```python
from build123d import *

# Parameters (mm, degrees)
SKETCH1_W           = 98
SKETCH1_H           = 65
BOSS_EXTRUDE1_DEPTH = 5
SKETCH2_W           = 16
SKETCH2_H           = 10
CUT_EXTRUDE1_DEPTH  = 15


with BuildPart() as part:
    # Sketch1 → Boss-Extrude1 (new body)
    with BuildSketch(Plane.XY):
        with Locations((49, -32.5)):
            Rectangle(SKETCH1_W, SKETCH1_H)
    extrude(amount=BOSS_EXTRUDE1_DEPTH)

    # Sketch2 → Cut-Extrude1 (cut)
    with BuildSketch(Plane.XY.offset(5)):
        Polygon((82, -45), (82, -40), (82, -35), (66, -35), (66, -45), align=None)
        with Locations((24, -40)):
            Rectangle(SKETCH2_W, SKETCH2_H)
    extrude(amount=-CUT_EXTRUDE1_DEPTH, mode=Mode.SUBTRACT)


solid = part.part
```
Design review of the part built by this model. Coordinates are the model's own, in mm. A direction names the side the tool comes from. Round coordinates to 2 decimals unless told otherwise and drop trailing zeros. Write each loop counter-clockwise with the first axis right and the second up, starting at its lowest first coordinate (ties: lowest second). Pieces come first, ordered by that corner, then holes. Notation, with made-up numbers: (-27, 27) -> (-10, 27) arc R28 cw to (-10, 51) -> close; hole circle Ø8 at (-13.75, -30.75). An arc over 180 degrees is marked (long way). Write item = value, one per line. Start each with the question number.
1) Tool access review of faces 1 (the face through (48, -32, 0)), 2 (the face through (24, -35, 3)): name each direction out of +Z, -Z, +X, -X, +Y, -Y from which nothing blocks a thin tool from reaching the whole face with its end or side.
2) Wall thickness on probe 1 along X at (y, z) = (-42.5, 2.5); probe 2 along Y at (x, z) = (80, 4.05): over which ranges is each line inside the solid? List them lowest first. Write a range as from..to.
3) Take a section at A-A, the plane y = -44. State the section outline as (x, z) points, plus the area to 3 significant figures.
4) Take a section at B-B, the plane x = 22.5. State the section outline as (y, z) points.
5) Mouldability with a two-part tool opening along X and no side actions: class faces 3 (the face through (74, -35, 3)), 4 (the face through (0, -33, 2)), 5 (the face through (48, -32, 5)), 6 (the face through (82, -40, 3)) as +X half, -X half, draft (parallel to the pull), parting line (faces both ways), or undercut.
6) Take a section at C-C, the plane z = 2.6. State the section outline as (x, y) points.
Results list:
q1.face_1 = -Z, +X, -X, +Y, -Y
q1.face_2 = +Z, -Z
q2.probe_1 = 0..16, 32..66, 82..98
q2.probe_2 = -65..-45, -35..0
q3.outline = (0, 0) -> (16, 0) -> (16, 5) -> (0, 5) -> close; (32, 0) -> (66, 0) -> (66, 5) -> (32, 5) -> close; (82, 0) -> (98, 0) -> (98, 5) -> (82, 5) -> close
q3.area = 330 mm²
q4.outline = (-65, 0) -> (-45, 0) -> (-45, 5) -> (-65, 5) -> close; (-35, 0) -> (0, 0) -> (0, 5) -> (-35, 5) -> close
q5.face_3 = undercut
q5.face_4 = -X half
q5.face_5 = draft
q5.face_6 = undercut
q6.outline = (0, -65) -> (98, -65) -> (98, 0) -> (0, 0) -> close; hole (16, -45) -> (32, -45) -> (32, -35) -> (16, -35) -> close; hole (66, -45) -> (82, -45) -> (82, -35) -> (66, -35) -> close
